Here's how the part is built. I have some questions about the finished solid (model axes, mm). Round coordinates to 2 decimals unless told otherwise and drop trailing zeros. Order: outer loops, then holes, each group sorted by start corner. A loop starts at its lowest first (then second) coordinate and runs counter-clockwise, first axis right, second up. Notation, with made-up numbers: (-27.5, -17) -> (14.5, -17) arc R25 ccw to (14.5, 11) -> close; hole circle Ø3 at (43, 1.5). An arc over 180 degrees is marked (long way). One line per item, written item: value.
```python
from build123d import *

# Parameters (mm, degrees)
SKETCH_1_W          = 250
SKETCH_1_H          = 110
EXTRUDE_1_DEPTH     = 4
SKETCH_3_R          = 2.1
CUT_EXTRUDE_1_DEPTH = 10
SKETCH_4_R          = 21
CUT_EXTRUDE_2_DEPTH = 10
SKETCH_5_R          = 2.05
CUT_EXTRUDE_3_DEPTH = 10
FILLET_1_R          = 2


with BuildPart() as part:
    # 草图1 → 凸台-拉伸1 (new body)
    with BuildSketch(Plane(origin=(0, 0, 0), x_dir=(1, 0, 0), z_dir=(0, 1, 0))):
        Rectangle(SKETCH_1_W, SKETCH_1_H)
    extrude(amount=EXTRUDE_1_DEPTH)

    # 草图3 → 切除-拉伸1 (cut)
    with BuildSketch(Plane(origin=(0, 4, 0), x_dir=(1, 0, 0), z_dir=(0, 1, 0))):
        with Locations(Location((-32.1, 0, 0), (0, 0, 270))):
            Circle(SKETCH_3_R)
        with Locations(Location((-16.05, 27.799415461, 0), (0, 0, 270))):
            Circle(SKETCH_3_R)
        with Locations(Location((16.05, 27.799415461, 0), (0, 0, 270))):
            Circle(SKETCH_3_R)
        with Locations(Location((32.1, 0, 0), (0, 0, 270))):
            Circle(SKETCH_3_R)
        with Locations(Location((16.05, -27.799415461, 0), (0, 0, 270))):
            Circle(SKETCH_3_R)
        with Locations(Location((-16.05, -27.799415461, 0), (0, 0, 270))):
            Circle(SKETCH_3_R)
    extrude(amount=-CUT_EXTRUDE_1_DEPTH, mode=Mode.SUBTRACT)

    # 草图4 → 切除-拉伸2 (cut)
    with BuildSketch(Plane(origin=(0, 4, 0), x_dir=(1, 0, 0), z_dir=(0, 1, 0))):
        with Locations(Location((0, 0, 0), (0, 0, 270))):
            Circle(SKETCH_4_R)
    extrude(amount=-CUT_EXTRUDE_2_DEPTH, mode=Mode.SUBTRACT)

    # 草图5 → 切除-拉伸3 (cut)
    with BuildSketch(Plane(origin=(0, 4, 0), x_dir=(1, 0, 0), z_dir=(0, 1, 0))):
        with Locations(Location((-110, 50, 0), (0, 0, 270))):
            Circle(SKETCH_5_R)
        with Locations(Location((-110, 40, 0), (0, 0, 270))):
            Circle(SKETCH_5_R)
        with Locations(Location((110, 40, 0), (0, 0, 270))):
            Circle(SKETCH_5_R)
        with Locations(Location((110, 50, 0), (0, 0, 270))):
            Circle(SKETCH_5_R)
        with Locations(Location((110, -50, 0), (0, 0, 270))):
            Circle(SKETCH_5_R)
        with Locations(Location((110, -40, 0), (0, 0, 270))):
            Circle(SKETCH_5_R)
        with Locations(Location((-110, -50, 0), (0, 0, 270))):
            Circle(SKETCH_5_R)
        with Locations(Location((-110, -40, 0), (0, 0, 270))):
            Circle(SKETCH_5_R)
    extrude(amount=-CUT_EXTRUDE_3_DEPTH, mode=Mode.SUBTRACT)

    # 圆角1
    fillet_1_edges = [part.edges().sort_by_distance(p)[0] for p in [
        (125, 2, 55),
        (-125, 2, 55),
        (-125, 2, -55),
        (125, 2, -55),
    ]]
    fillet(fillet_1_edges, radius=FILLET_1_R)


solid = part.part
```
Q1. I want a section at C-C on x = 3.5. Write out the boundary of the cut face in (y, z).
Answers:
outline: (0, -55) -> (4, -55) -> (4, -20.71) -> (0, -20.71) -> close; (0, 20.71) -> (4, 20.71) -> (4, 55) -> (0, 55) -> close
Q2. I want a section at B-B on z = 4.5. Write out the boundary of the cut face in (x, y), then the cut area to 3 significant figures.
Answers:
outline: (-125, 0) -> (-20.51, 0) -> (-20.51, 4) -> (-125, 4) -> close; (20.51, 0) -> (125, 0) -> (125, 4) -> (20.51, 4) -> close
area: 836 mm2
Q3. For P1, Ø3.5, axis at x = 110, z = -50, coming from the +Y side, with a flat end and sliding along its axis, tell me the tip position at first contact or that it passes through.
Answers:
P1: through
Q4. I need wall thicknesses on line 1 along X through (y, z) = (1.75, -40); line 2 along X through (y, z) = (2.1, -15); line 3 along Z through (x, y) = (30.5, 1.65). Which ranges of each line are inside material? Lowest first, please.
Answers:
line 1: -125 to -112.05, -107.95 to 107.95, 112.05 to 125
line 2: -125 to -14.7, 14.7 to 125
line 3: -55 to -1.36, 1.36 to 55
Q5. If we mould it in two halves opening along Z, with no side actions, what happens to faces 1 (the face through (-2, 0, -25)), 2 (the face through (112.033, 2.028, 39.733))? For each: pulls with the +Z half, pulls with the -Z half, needs draft (parallel to the pull), parting line crosses it, or undercut.
Answers:
face 1: needs draft
face 2: undercut
Q6. I want a section at A-A on y = 1.55. Give the number of separate pieces and of enclosed holes in the cut face, then the cut area to 3 significant figures.
Answers:
separate pieces: 1
enclosed holes: 15
area: 25,900 mm2
